from build123d import *

# Parameters (mm, degrees)
BOX_W        = 8
BOX_H        = 10
BOX_DEPTH    = 7.5
SKETCH001_W  = 32
SKETCH001_H  = 43
PAD001_DEPTH = 7.5
SKETCH_W     = 22
SKETCH_H     = 33
SKETCH_W_2   = 12
SKETCH_H_2   = 23
PAD_DEPTH    = 15


with BuildPart() as cube:
    # Box → Box (new body)
    with BuildSketch(Plane(origin=(-4, 8, 7.5), x_dir=(1, 0, 0), z_dir=(0, 0, 1))):
        with Locations((4, 5)):
            Rectangle(BOX_W, BOX_H)
    extrude(amount=BOX_DEPTH)


with BuildPart() as body001:
    # Sketch001 → Pad001 (new body)
    with BuildSketch(Plane.XY):
        Rectangle(SKETCH001_W, SKETCH001_H)
    extrude(amount=PAD001_DEPTH)


with BuildPart() as cut:
    # Sketch → Pad (new body)
    with BuildSketch(Plane.XY):
        Rectangle(SKETCH_W, SKETCH_H)
        Rectangle(SKETCH_W_2, SKETCH_H_2, mode=Mode.SUBTRACT)
    extrude(amount=PAD_DEPTH)

    # Fusion: union Body001
    add(body001.part)

    # Cut: cut Cube
    add(cube.part, mode=Mode.SUBTRACT)


solid = cut.part
Geometry check sheet. Reference: the model listing, model coordinates, mm. A direction names the side the tool comes from. Round coordinates to 2 decimals unless told otherwise and drop trailing zeros. Loops run counter-clockwise (first coordinate to the right, second up) from the corner with the lowest first, then second, coordinate; pieces in that order, holes last. Notation, with made-up numbers: (-17.75, 75) - (30.25, 75) arc R21 cw to (30.25, 109) - close; hole circle Ø5 at (-19, -30). An arc over 180 degrees is marked (long way). Answer as CSV lines item,"result".
(1) Depth check by flat-ended pin: pin 1 Ø12 at (x, y) = (-7, -6) entering from -Z; pin 2 Ø2 at (y, z) = (4, 10) entering from -X; pin 3 Ø1 at (x, y) = (-12.5, 15.5) entering from +Z; pin 4 Ø4 at (y, z) = (16, 10.5) entering from +X. Enter the tip coordinate at first touch or a pass-through.
Output values:
pin 1,"stops at z = 0"
pin 2,"stops at x = -11"
pin 3,"stops at z = 7.5"
pin 4,"stops at x = 11"
(2) Cross-section at A-A, the plane y = 13. Enter the section's corners in (x, z).
Output values:
outline,"(-16, 0) - (16, 0) - (16, 7.5) - (11, 7.5) - (11, 15) - (4, 15) - (4, 7.5) - (-4, 7.5) - (-4, 15) - (-11, 15) - (-11, 7.5) - (-16, 7.5) - close"
(3) Cross-section at D-D, the plane x = 0.5. Enter the section's corners in (y, z), and give its area (3 significant figures).
Output values:
outline,"(-21.5, 0) - (21.5, 0) - (21.5, 7.5) - (-11.5, 7.5) - (-11.5, 15) - (-16.5, 15) - (-16.5, 7.5) - (-21.5, 7.5) - close"
area,"360 mm²"
(4) Set-up check for faces 1 (the face through (4, 14, 11)), 2 (the face through (11, 0, 11)), 3 (the face through (7, 16.5, 11)), 4 (the face through (6, 0, 11)), 5 (the face through (0, -16.5, 11)): record each of +Z, -Z, +X, -X, +Y, -Y from which the full face is reachable in a straight line by a thin tool's end or side.
Output values:
face 1,"+Z, +Y"
face 2,"+Z, +X, +Y, -Y"
face 3,"+Z, +X, -X, +Y"
face 4,"+Z"
face 5,"+Z, +X, -X, -Y"
(5) Cross-section at C-C, the plane x = -8. Enter the section's corners in (y, z), and give its area (3 significant figures).
Output values:
outline,"(-21.5, 0) - (21.5, 0) - (21.5, 7.5) - (16.5, 7.5) - (16.5, 15) - (-16.5, 15) - (-16.5, 7.5) - (-21.5, 7.5) - close"
area,"570 mm²"
(6) Cross-section at B-B, the plane z = 13. Enter the section's corners in (x, y).
Output values:
outline,"(-11, -16.5) - (11, -16.5) - (11, 16.5) - (4, 16.5) - (4, 11.5) - (6, 11.5) - (6, -11.5) - (-6, -11.5) - (-6, 11.5) - (-4, 11.5) - (-4, 16.5) - (-11, 16.5) - close"
(7) Material ranges on line 1 along X through (y, z) = (16, 11); line 2 along X through (y, z) = (-3.5, 11.5); line 3 along Z through (x, y) = (-12.5, -17.5), recorded low to high.
Output values:
line 1,"x = -11 to -4, 4 to 11"
line 2,"x = -11 to -6, 6 to 11"
line 3,"z = 0 to 7.5"
(8) Release check for a two-part mould opening along X. For faces 6 (the face through (-7, 0, 15)), 7 (the face through (-11, 0, 11)), 8 (the face through (0, -11.5, 11)) record: released by +X, released by -X, zero draft, split by the parting line, or undercut.
Output values:
face 6,"zero draft"
face 7,"released by -X"
face 8,"undercut"
